Geometry: see drawing. Coordinates: mm, zero at the bounding-box minimum. A direction names the side the tool comes from. Round coordinates to 2 decimals unless told otherwise and drop trailing zeros. Order: outer loops, then holes, each group sorted by start corner. A loop starts at its lowest first (then second) coordinate and runs counter-clockwise, first axis right, second up. Notation, with made-up numbers: (59.25, -9.5) -> (92.25, -9.5) arc R12 cw to (92.25, -4.5) -> close; hole circle Ø3 at (-23, 41.5). An arc over 180 degrees is marked (long way). Put each result on its own line as item: value.
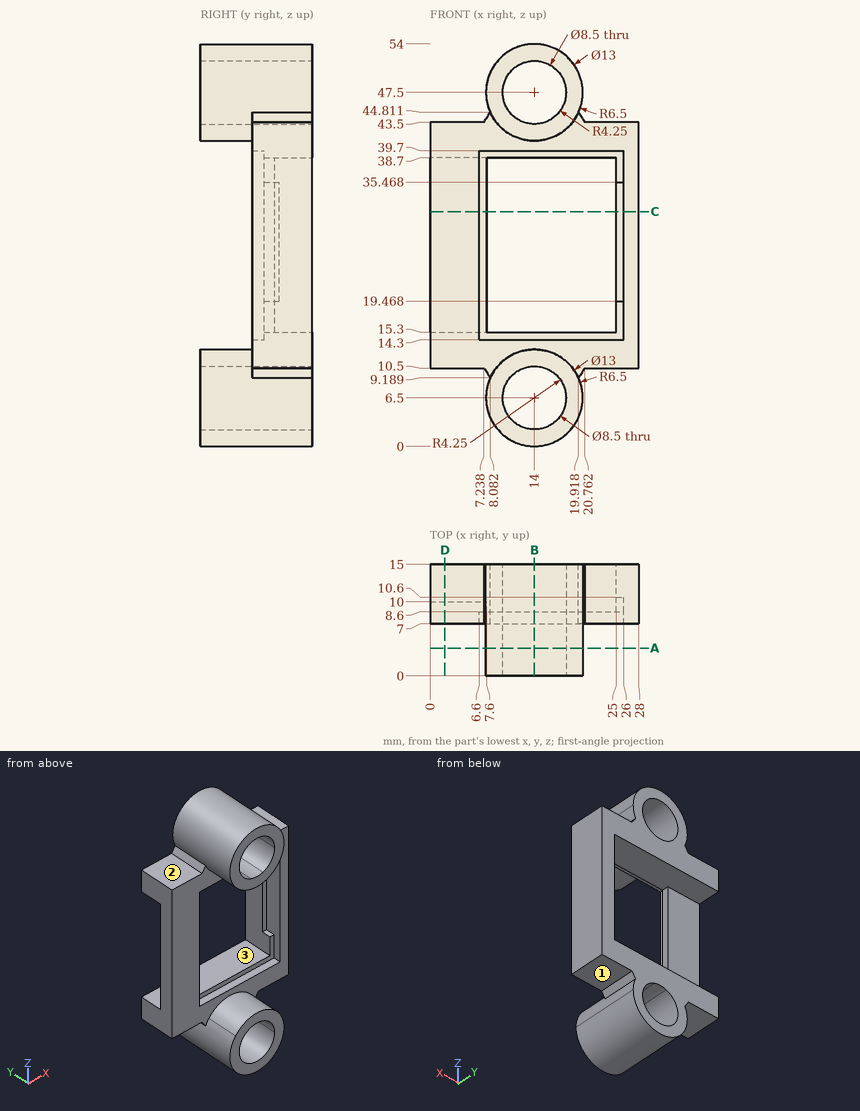
1. Cut plane C-C on z = 31.5. Return loops of the section in (x, y), and give its area (3 significant figures).
Ans:
outline: (0, 7) -> (6.6, 7) -> (6.6, 8.6) -> (7.6, 8.6) -> (7.6, 10) -> (0, 10) -> close; (25, 10.6) -> (26, 10.6) -> (26, 7) -> (28, 7) -> (28, 15) -> (25, 15) -> close
area: 41.6 mm²
2. Material intervals for probe 1 along Z at (x, y) = (14, 11); probe 2 along Z at (x, y) = (14, 6.5); probe 3 along X at (y, z) = (9.25, 26.5), sorted ascending.
Ans:
probe 1: 0 to 2.25, 10.75 to 15.3, 38.7 to 43.25, 51.75 to 54
probe 2: 0 to 2.25, 10.75 to 13, 41 to 43.25, 51.75 to 54
probe 3: 0 to 7.6, 26 to 28
3. Set-up query: the marked faces 1, 2 and 3. Return all of +Z, -Z, +X, -X, +Y, -Y with unobstructed straight access to the full face (end or side cutting, diameter ignored); none if empty.
Ans:
face 1: -Z, +X, +Y, -Y
face 2: +Z, -X, +Y, -Y
face 3: +Y
4. Cut plane A-A on y = 3.75. Return loops of the section in (x, z), and give its area (3 significant figures).
Ans:
outline: circle Ø13 at (14, 6.5); circle Ø13 at (14, 47.5); hole circle Ø8.5 at (14, 6.5); hole circle Ø8.5 at (14, 47.5)
area: 152 mm²
5. Cut plane D-D on x = 2. Return loops of the section in (y, z), and give its area (3 significant figures).
Ans:
outline: (7, 10.5) -> (15, 10.5) -> (15, 15.3) -> (10, 15.3) -> (10, 38.7) -> (15, 38.7) -> (15, 43.5) -> (7, 43.5) -> close
area: 147 mm²
6. Cut plane B-B on x = 14. Return loops of the section in (y, z).
Ans:
outline: (0, 0) -> (15, 0) -> (15, 2.25) -> (0, 2.25) -> close; (0, 10.75) -> (15, 10.75) -> (15, 15.3) -> (8.6, 15.3) -> (8.6, 14.3) -> (7, 14.3) -> (7, 13) -> (0, 13) -> close; (0, 41) -> (7, 41) -> (7, 39.7) -> (8.6, 39.7) -> (8.6, 38.7) -> (15, 38.7) -> (15, 43.25) -> (0, 43.25) -> close; (0, 51.75) -> (15, 51.75) -> (15, 54) -> (0, 54) -> close
7. Contact query for flat-ended pins moving along their axis: P1, Ø8, axis at y = 6.5, z = 25, coming from the +X side; P2, Ø1, axis at x = 17, y = 5, coming from the -Z side; P3, Ø3, axis at x = 3, y = 7, coming from the +Z side; P4, Ø8.5, axis at x = 5, z = 29.5, coming from the +Y side. Output: stop coordinate, or through.
Ans:
P1: x = 28
P2: z = 0.5
P3: z = 43.5
P4: y = 10
